```python
from build123d import *

# Parameters (mm, degrees)
PAD_DEPTH    = 1
SKETCH002_R  = 5
PAD001_DEPTH = 10


with BuildPart() as part:
    # Sketch → Pad (new body)
    with BuildSketch(Plane.XY):
        with BuildLine():
            Line((-26.647359, 7.054149), (-26.647359, 7.041504))
            ThreePointArc((-26.647359, 7.041504), (-24.745405, 2.449781), (-20.153681, 0.547826))
            Line((-20.153681, 0.547826), (-7.141037, 0.547826))
            ThreePointArc((-7.141037, 0.547826), (-2.549313, 2.449781), (-0.647359, 7.041504))
            Line((-0.647359, 7.041504), (-0.647359, 7.054149))
            ThreePointArc((-0.647359, 7.054149), (-2.549313, 11.645872), (-7.141037, 13.547826))
            Line((-7.141037, 13.547826), (-20.153681, 13.547826))
            ThreePointArc((-20.153681, 13.547826), (-24.745405, 11.645872), (-26.647359, 7.054149))
        make_face()
    extrude(amount=PAD_DEPTH)

    # Sketch002 (on Face10 of Pad) → Pad001 (join)
    with BuildSketch(Plane.XY.offset(1)):
        with Locations((-20.153681, 7.054149)):
            Circle(SKETCH002_R)
        with Locations((-7.141037, 7.041504)):
            Circle(SKETCH002_R)
    extrude(amount=PAD001_DEPTH)


solid = part.part
```
Here's how the part is built. I have some questions about the finished solid (model axes, mm). A direction names the side the tool comes from. Give positions to 0.01 mm unless a question says otherwise; leave off trailing zeros. Loops run counter-clockwise (first coordinate to the right, second up) from the corner with the lowest first, then second, coordinate; pieces in that order, holes last. Notation, with made-up numbers: M 72.25,29 L 113.25,29 A7 cw 113.25,38 Z; hole C 26.5,44 d7. An arc over 180 degrees is marked long. Return JSON: item names as keys, results as strings.
Item 1: Imagine slicing it at D-D on x = -11. List the corners of the cut face in (y, z) for me, then the cut area to 3 significant figures.
A:
{"outline": "M 0.55,0 L 13.55,0 L 13.55,1 L 10.22,1 L 10.22,11 L 3.86,11 L 3.86,1 L 0.55,1 Z", "area": "76.6 mm^2"}
Item 2: Please list where these lines run through material, in increasing order: line 1 (Z direction, x = -19.75, y = 12.5); line 2 (X direction, y = 11.25, z = 9.75); line 3 (X direction, y = 5.25, z = 6.5).
A:
{"line 1": "z = 0 to 1", "line 2": "x = -22.87 to -17.43, -9.84 to -4.44", "line 3": "x = -24.82 to -15.49, -11.81 to -2.47"}
Item 3: Imagine slicing it at A-A on z = 9.5. List the corners of the cut face in (x, y) for me, then the cut area to 3 significant figures.
A:
{"outline": "C -20.15,7.05 d10; C -7.14,7.04 d10", "area": "157 mm^2"}
Item 4: Thinking about a two-plate mould opening in X: for faces 1 (the cylindrical face through (-24.796, 2.501, 0.493)), 2 (the flat face through (-7, 7, 11)), 3 (the flat face through (-14, 7, 1)), which applies, released by +X, released by -X, zero draft, split by the parting line, or undercut?
A:
{"face 1": "released by -X", "face 2": "zero draft", "face 3": "undercut"}
Item 5: Imagine slicing it at C-C on x = -19.5. List the corners of the cut face in (y, z) for me.
A:
{"outline": "M 0.55,0 L 13.55,0 L 13.55,1 L 12.01,1 L 12.01,11 L 2.1,11 L 2.1,1 L 0.55,1 Z"}
Item 6: Imagine slicing it at B-B on y = 7.5. List the corners of the cut face in (x, z) for me.
A:
{"outline": "M -26.63,0 L -0.66,0 L -0.66,1 L -2.16,1 L -2.16,11 L -12.12,11 L -12.12,1 L -15.17,1 L -15.17,11 L -25.13,11 L -25.13,1 L -26.63,1 Z"}
Item 7: On a 3-axis mill with a long thin cutter (end or side, diameter ignored), from which of +Z, -Z, +X, -X, +Y, -Y can I reach the whole of each face in a straight line? I mean faces 4 (the cylindrical face through (-2.499, 11.595, 0.493)), 5 (the cylindrical face through (-11.11, 4, 5.93)). Say none if no direction works.
A:
{"face 4": "+Z, -Z, +X, +Y", "face 5": "+Z"}
Item 8: I'm going to push flat-ended pins straight in: pin 1 Ø1 at (x, z) = (-5, 5) entering from -Y; pin 2 Ø1 at (x, z) = (-19, 3.5) entering from -Y; pin 3 Ø5 at (y, z) = (3, 10) entering from -X. Where does each tip first touch, or does it pass through?
A:
{"pin 1": "stops at y = 2.32", "pin 2": "stops at y = 2.1", "pin 3": "stops at x = -24.91"}
